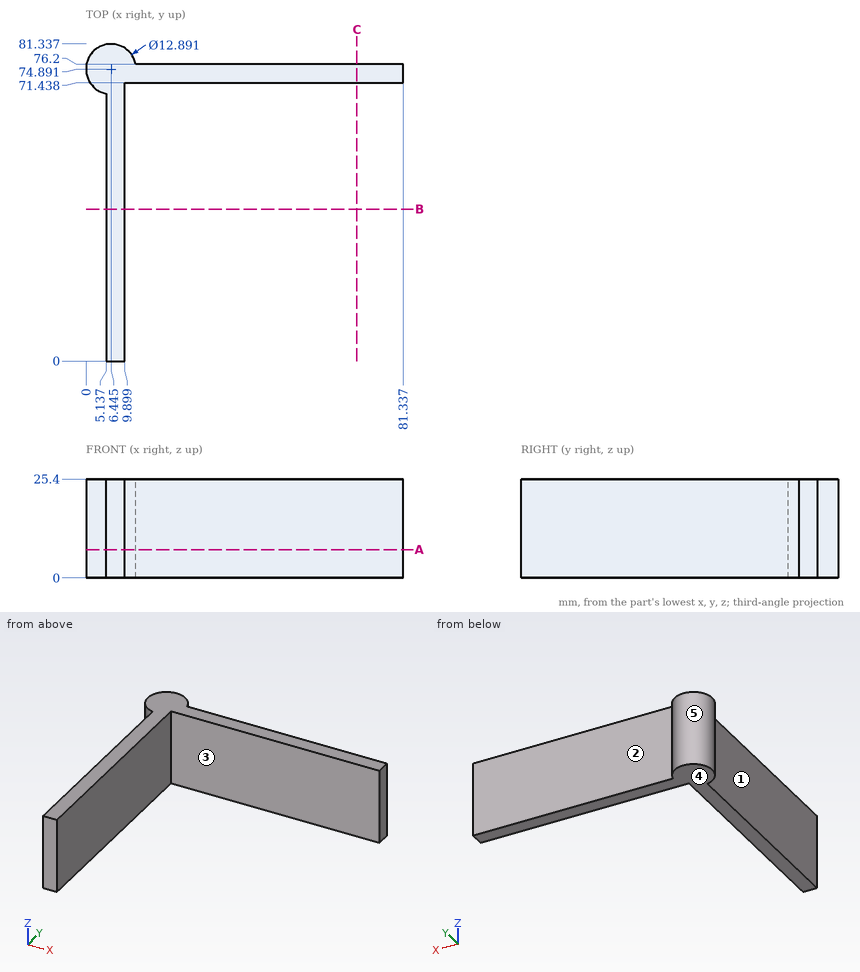
Verification items for this drawing (mm, ordinates from the low corner). A direction names the side the tool comes from. Round coordinates to 2 decimals unless told otherwise and drop trailing zeros. Loops run counter-clockwise (first coordinate to the right, second up) from the corner with the lowest first, then second, coordinate; pieces in that order, holes last. Notation, with made-up numbers: (40.25, 25) -> (62.25, 25) arc R22 ccw to (62.25, 34) -> close; hole circle Ø7 at (-19.75, 79.5). An arc over 180 degrees is marked (long way). Answer in a Markdown table with one row per item.
Q1. Sectioned sample at A-A on z = 7.25. Enter the section's corners in (x, y) (1 decimal).
Data:
| item | result |
|---|---|
| outline | (5.1, 0) -> (9.9, 0) -> (9.9, 71.4) -> (81.3, 71.4) -> (81.3, 76.2) -> (12.8, 76.2) arc R6.4 ccw (long way) to (5.1, 68.6) -> close |
Q2. Go/stop test with flat-tipped pins: P1, Ø3, axis at y = 11, z = 10, coming from the -X side; P2, Ø6, axis at y = 68, z = 17, coming from the +X side; P3, Ø5, axis at x = 55.5, z = 16.5, coming from the +Y side; P4, Ø12, axis at x = 48, y = 67, coming from the +Z side. Record where each tip stops, or that it passes through.
Data:
| item | result |
|---|---|
| P1 | stops at x = 5.14 |
| P2 | stops at x = 9.9 |
| P3 | stops at y = 76.2 |
| P4 | stops at z = 25.4 |
Q3. Sectioned sample at B-B on y = 39. Enter the section's corners in (x, z).
Data:
| item | result |
|---|---|
| outline | (5.14, 0) -> (9.9, 0) -> (9.9, 25.4) -> (5.14, 25.4) -> close |
Q4. Thickness scan on L1, parallel to X at y = 61, z = 2; L2, parallel to Y at x = 31.5, z = 1.5; L3, parallel to Y at x = 12, z = 10.5 (1 decimal). Record the ranges inside material, lowest first.
Data:
| item | result |
|---|---|
| L1 | x = 5.14 to 9.9 |
| L2 | y = 71.44 to 76.2 |
| L3 | y = 71.4 to 78.2 |
Q5. Sectioned sample at C-C on x = 69.5. Enter the section's corners in (y, z).
Data:
| item | result |
|---|---|
| outline | (71.44, 0) -> (76.2, 0) -> (76.2, 25.4) -> (71.44, 25.4) -> close |
Q6. Set-up check for the marked faces 1, 2, 3, 4 and 5: record each of +Z, -Z, +X, -X, +Y, -Y from which the full face is reachable in a straight line by a thin tool's end or side.
Data:
| item | result |
|---|---|
| face 1 | +Z, -Z, -X, -Y |
| face 2 | +Z, -Z, +X, +Y |
| face 3 | +Z, -Z, +X, -Y |
| face 4 | -Z, +X, -X, +Y, -Y |
| face 5 | +Z, -Z |
